Design review of the part shown in the three views and the two pictorial views. Dimensions are in mm from the part's minimum x, y and z. A direction names the side the tool comes from. Coordinates: 2 decimals unless noted, no trailing zeros. Write each loop counter-clockwise with the first axis right and the second up, starting at its lowest first coordinate (ties: lowest second). Pieces come first, ordered by that corner, then holes.
Q1. For pin 1 Ø3 at (x, y) = (12, 21) entering from -Z (1 decimal); pin 2 Ø1.5 at (x, z) = (13.5, 9) entering from +Y; pin 3 Ø1.5 at (x, y) = (17.5, 13.5) entering from -Z; pin 4 Ø1 at (x, z) = (16.5, 9.5) entering from -Y, all flat-tipped, find the tip position at first contact; note any pin that passes through.
Q2. Take a section at A-A, the plane y = 12. Write out the cut boundary in (x, z), plus the area to 3 significant figures.
Q3. Take a section at D-D, the plane x = 14.5. Write out the cut boundary in (y, z), plus the area to 3 significant figures.
Q4. Take a section at C-C, the plane z = 1.5. Write out the cut boundary in (x, y).
Q5. For the marked faces 1 and 2, list the 3-axis set-ups (+Z, -Z, +X, -X, +Y, -Y) from which the entire face can be reached by the end or side of a thin tool; tool diameter is ignored.
Q6. For L1, parallel to Y at x = 12, z = 0.7; L2, parallel to Y at x = 21, z = 0.8; L3, parallel to Y at x = 12, z = 8.25, list the stretches that pass through material, from the lowest coordinate up.
Q7. The part is to be moulded in two halves that separate along X. For the marked faces 3, 4 and 5, say which applies: released by +X, released by -X, zero draft, split by the parting line, or undercut.
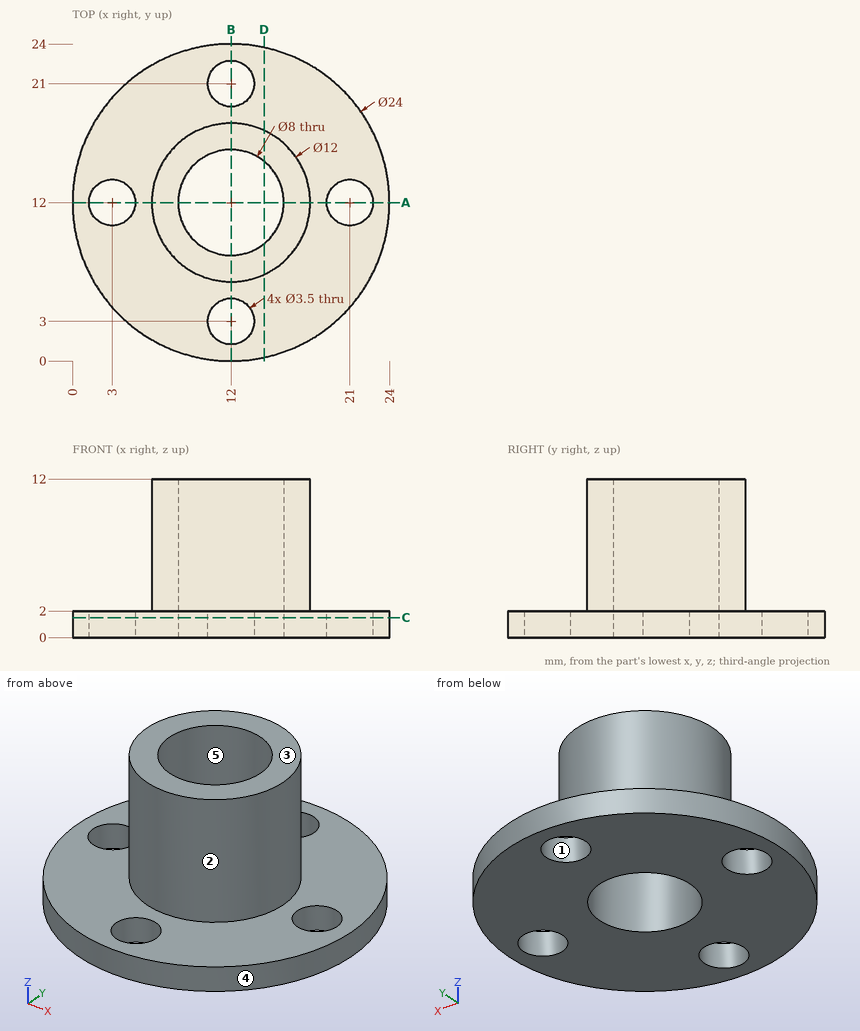
Responses:
1. pin 1: passes through
1. pin 2: stops at y = 17.95
1. pin 3: stops at z = 0
1. pin 4: stops at y = 7.53
2. outline: (0, 0) - (1.25, 0) - (1.25, 2) - (0, 2) - close; (4.75, 0) - (8, 0) - (8, 12) - (6, 12) - (6, 2) - (4.75, 2) - close; (16, 0) - (19.25, 0) - (19.25, 2) - (18, 2) - (18, 12) - (16, 12) - close; (22.75, 0) - (24, 0) - (24, 2) - (22.75, 2) - close
2. area: 58.0 mm2
3. outline: (0.26, 0) - (8.88, 0) - (8.88, 12) - (6.55, 12) - (6.55, 2) - (0.26, 2) - close; (15.12, 0) - (23.74, 0) - (23.74, 2) - (17.45, 2) - (17.45, 12) - (15.12, 12) - close
3. area: 81.1 mm2
4. outline: circle Ø24 at (12, 12); hole circle Ø3.5 at (3, 12); hole circle Ø8 at (12, 12); hole circle Ø3.5 at (12, 3); hole circle Ø3.5 at (12, 21); hole circle Ø3.5 at (21, 12)
5. face 1: +Z, -Z
5. face 2: +Z
6. L1: y = 0 to 1.25, 4.75 to 8, 16 to 19.25, 22.75 to 24
6. L2: y = 4.06 to 10.25, 13.75 to 19.94
6. L3: y = 6 to 8, 16 to 18
7. face 3: zero draft
7. face 4: split by the parting line
7. face 5: undercut
